Part model, mm, in its own coordinate system. A direction names the side the tool comes from. Give positions to 0.01 mm unless a question says otherwise; leave off trailing zeros. Order: outer loops, then holes, each group sorted by start corner. A loop starts at its lowest first (then second) coordinate and runs counter-clockwise, first axis right, second up. Notation, with made-up numbers: (-32, 52) -> (27, 52) arc R17 cw to (27, 63) -> close; hole circle Ø1 at (-5.5, 56). An arc over 180 degrees is marked (long way). Write item = value, one per line. Start each with the question number.
(1) Saw through at B-B, the plane x = -13. List the corners of the cut face in (y, z), then the cut area to 3 significant figures.
(2) Flat gauge pins, fed straight in: pin 1 (5 mm diameter, centred on x = -17.5, z = 482, fed in from +Y); pin 2 (1.9 mm diameter, centred on y = 2.5, z = 446, fed in from -X); pin 3 (3 mm diameter, centred on x = -16, z = 521, fed in from +Y). Where does each tip first touch, or does it go through?
(3) Probe line 1 along X through (y, z) = (13.75, 164.5); line 2 along X through (y, z) = (14.75, 482.5); line 3 along X through (y, z) = (3.75, 25.4). List the from-to ranges inside material, lowest first. Write a range as from..to.
(4) Which spindle directions (+Z, -Z, +X, -X, +Y, -Y) get a long thin tool onto all of the face, cutting with end or side? Do faces 1 (the flat face through (13, 0, 301)), 2 (the flat face through (-9, 7.5, 301)). Say none if no direction does.
(5) Saw through at A-A, the plane z = 192. List the corners of the cut face in (x, y), then the cut area to 3 significant figures.
(6) Two-plate mould, pull along X, no slides. Class faces 3 (the cylindrical face through (-34.27, 20.02, 300.53)), 4 (the cylindrical face through (34.671, 19.643, 300.533)): pulls with the +X half, pulls with the -X half, needs draft (parallel to the pull), parting line crosses it, or undercut.
from build123d import *

# Parameters (mm, degrees)
MODEL_R                           = 3.999999997
BOSS_EXTRUDE1_DEPTH               = 609.6
F_3_8_16_TAPPED_HOLE1_D           = 7.9375
F_3_8_16_TAPPED_HOLE1_CSINK_D     = 10.16
F_3_8_16_TAPPED_HOLE1_CSINK_ANGLE = 90
CUT_EXTRUDE1_DEPTH                = 612.11795915
TAP_DRILL_FOR_0_80_TAP1_D         = 1.19126


with BuildPart() as part:
    # Model → Boss-Extrude1 (new body)
    with BuildSketch(Plane.XY):
        with BuildLine():
            Line((-18.843780991, 7.981867858), (-20.966888929, 12.534890876))
            ThreePointArc((-20.966888929, 12.534890876), (-21.047789267, 12.798072701), (-21.053849819, 13.07334131))
            ThreePointArc((-21.053849819, 13.07334131), (-34.474612004, 19.833405747), (-28.578947374, 6.011088019))
            ThreePointArc((-28.578947374, 6.011088019), (-27.4676292, 5.601381399), (-27.000000001, 4.513167022))
            Line((-27.000000001, 4.513167022), (-27.000000001, 0.700000022))
            Line((-27.000000001, 0.700000022), (-26.500000001, 0.200000022))
            Line((-26.500000001, 0.200000022), (-20.200001001, 0.200000022))
            Line((-20.200001001, 0.200000022), (-20.000000979, 0))
            Line((-20.000000979, 0), (-6.000000502, 0))
            Line((-6.000000502, 0), (-5.80000048, 0.200000022))
            Line((-5.80000048, 0.200000022), (5.80000048, 0.200000022))
            Line((5.80000048, 0.200000022), (6.000000502, 0))
            Line((6.000000502, 0), (20.000000979, 0))
            Line((20.000000979, 0), (20.200001001, 0.200000022))
            Line((20.200001001, 0.200000022), (26.500000001, 0.200000022))
            Line((26.500000001, 0.200000022), (27.000000001, 0.700000022))
            Line((27.000000001, 0.700000022), (27.000000001, 4.513167022))
            ThreePointArc((27.000000001, 4.513167022), (27.4676292, 5.601381399), (28.578947374, 6.011088019))
            ThreePointArc((28.578947374, 6.011088019), (34.474612004, 19.833405747), (21.053849819, 13.07334131))
            ThreePointArc((21.053849819, 13.07334131), (21.047789267, 12.798072701), (20.966888929, 12.534890876))
            Line((20.966888929, 12.534890876), (18.843780991, 7.981867858))
            ThreePointArc((18.843780991, 7.981867858), (18.479330527, 7.628755749), (17.98848008, 7.499999621))
            Line((17.98848008, 7.499999621), (0.500000254, 7.499999621))
            Line((0.500000254, 7.499999621), (0, 7.211324621))
            Line((0, 7.211324621), (-0.500000254, 7.499999621))
            Line((-0.500000254, 7.499999621), (-17.98848008, 7.499999621))
            ThreePointArc((-17.98848008, 7.499999621), (-18.479330527, 7.628755749), (-18.843780991, 7.981867858))
        make_face()
        with Locations(Location((-29.000000026, 13.999999962, 0), (0, 0, 180))):
            Circle(MODEL_R, mode=Mode.SUBTRACT)
        with Locations(Location((29.000000026, 13.999999962, 0), (0, 0, 180))):
            Circle(MODEL_R, mode=Mode.SUBTRACT)
    extrude(amount=BOSS_EXTRUDE1_DEPTH)

    # 3/8-16 Tapped Hole1 (through all)
    with Locations(Plane(origin=(0, 7.499999621, 0), x_dir=(1, 0, 0), z_dir=(0, 1, 0))):
        with Locations((0, -25.4), (0, -127), (0, -228.6), (0, -330.2), (0, -431.8), (0, -533.4), (0, -635), (0, -736.6), (0, -838.2), (0, -939.8), (0, -1041.4), (0, -1143), (0, -1244.6), (0, -1346.2), (0, -1447.8), (0, -1549.4), (0, -1651), (0, -1752.6), (0, -1854.2), (0, -1955.8)):
            CounterSinkHole(F_3_8_16_TAPPED_HOLE1_D / 2, F_3_8_16_TAPPED_HOLE1_CSINK_D / 2, counter_sink_angle=F_3_8_16_TAPPED_HOLE1_CSINK_ANGLE)

    # Sketch3 → Cut-Extrude1 (cut, through all)
    with BuildSketch(Plane(origin=(0, 0, 0), x_dir=(-1, 0, 0), z_dir=(0, 0, -1))):
        Polygon((-17.98848008, 7.499999621), (-21.053849819, 7.499999621), (-21.053849819, 13.07334131), align=None)
    extrude(amount=-CUT_EXTRUDE1_DEPTH, mode=Mode.SUBTRACT)

    # Tap Drill for #0-80 Tap1 (through all)
    with Locations(Plane(origin=(0, 7.499999621, 0), x_dir=(1, 0, 0), z_dir=(0, 1, 0))):
        with Locations((19.402849819, -3.309755123), (19.402849819, -103.055555123), (19.402849819, -202.801355123), (19.402849819, -302.547155123), (19.402849819, -402.292955123), (19.402849819, -502.038755123), (19.402849819, -601.784555123), (19.402849819, -701.530355123), (19.402849819, -801.276155123), (19.402849819, -901.021955123)):
            Hole(TAP_DRILL_FOR_0_80_TAP1_D / 2)


solid = part.part
Results list:
q1.outline = (0, 0) -> (7.5, 0) -> (7.5, 609.6) -> (0, 609.6) -> close
q1.area = 4,570 mm^2
q2.pin_1 = 10.46
q2.pin_2 = -27
q2.pin_3 = 7.5
q3.line_1 = -37..-32.99, -25.01..-21, 21..25.01, 32.99..37
q3.line_2 = -36.96..-32.93, -25.07..-21.04, 21.04..25.07, 32.93..36.96
q3.line_3 = -27..-3.97, 3.97..27
q4.face_1 = +Z, -Z, +X, -X, -Y
q4.face_2 = +Z, -Z, +Y
q5.outline = (-28.58, 6.01) arc R1.5 cw to (-27, 4.51) -> (-27, 0.7) -> (-26.5, 0.2) -> (-20.2, 0.2) -> (-20, 0) -> (-6, 0) -> (-5.8, 0.2) -> (5.8, 0.2) -> (6, 0) -> (20, 0) -> (20.2, 0.2) -> (26.5, 0.2) -> (27, 0.7) -> (27, 4.51) arc R1.5 cw to (28.58, 6.01) arc R8 ccw (long way) to (21.05, 13.07) arc R1 cw to (21.05, 12.84) -> (21.05, 7.5) -> (0.5, 7.5) -> (0, 7.21) -> (-0.5, 7.5) -> (-17.99, 7.5) arc R1 cw to (-18.84, 7.98) -> (-20.97, 12.53) arc R1 cw to (-21.05, 13.07) arc R8 ccw (long way) to start; hole circle Ø8 at (-29, 14); hole circle Ø8 at (29, 14)
q5.area = 717 mm^2
q6.face_3 = undercut
q6.face_4 = undercut
